Work out the finished part from the listing and answer in its coordinate system (mm). Face numbers are marked on the shaded views. Round coordinates to 2 decimals unless told otherwise and drop trailing zeros. Loops run counter-clockwise (first coordinate to the right, second up) from the corner with the lowest first, then second, coordinate; pieces in that order, holes last. Notation, with made-up numbers: (47, 54.25) -> (86, 54.25) arc R33 ccw to (86, 83.25) -> close; hole circle Ø1 at (27.5, 79). An arc over 180 degrees is marked (long way). Use one line per item in the form item = value.
```python
from build123d import *

# Parameters (mm, degrees)
F0_W     = 25.4
F0_H     = 25.4
F0_W_2   = 22.225
F0_H_2   = 22.225
F1_DEPTH = 292.1
F3_DEPTH = 25.401
F5_DEPTH = 25.401


with BuildPart() as f1:
    # F0 (on Front) → F1 (new body, symmetric)
    with BuildSketch(Plane.XZ):
        Rectangle(F0_W, F0_H)
        Rectangle(F0_W_2, F0_H_2, mode=Mode.SUBTRACT)
    extrude(amount=F1_DEPTH, both=True)

    # F2 (on face) → F3 (cut, through all)
    with BuildSketch(Plane.XY.offset(12.7)):
        Polygon((12.7, 292.1), (-12.7, 292.1), (-12.7, 287.621295), align=None)
    extrude(amount=-F3_DEPTH, mode=Mode.SUBTRACT)

    # F4 (on face) → F5 (cut, through all)
    with BuildSketch(Plane.XY.offset(12.7)):
        Polygon((12.7, -287.621295), (-12.7, -292.1), (12.7, -292.1), align=None)
    extrude(amount=-F5_DEPTH, mode=Mode.SUBTRACT)


solid = f1.part
```
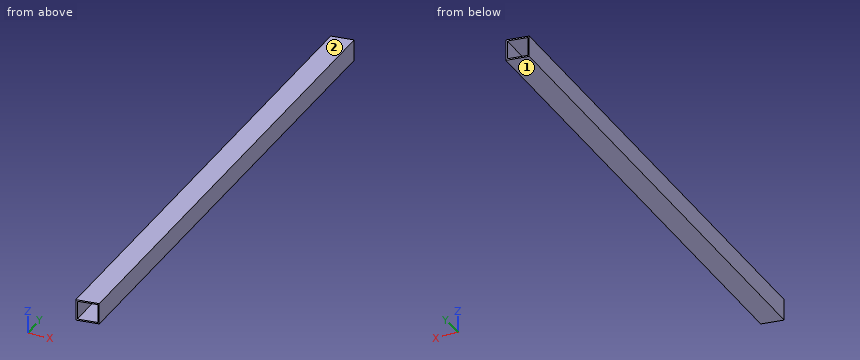
(1) Consider L1, parallel to Z at x = -10.5, y = -87. Determine where the line is inside the solid, lowest interval first.
Completed:
L1 = -12.7 to -11.11, 11.11 to 12.7
(2) For a pull along Z with two mould halves and no side action, classify the marked faces 1 and 2 as +Z half, -Z half, draft (parallel to the pull), parting line (faces both ways), or undercut.
Completed:
face_1 = -Z half
face_2 = +Z half
(3) Find section A-A, the plane y = 118.5. Write down the section's boundary in (x, z), then the cut area to 3 significant figures.
Completed:
outline = (-12.7, -12.7) -> (12.7, -12.7) -> (12.7, 12.7) -> (-12.7, 12.7) -> close; hole (-11.11, -11.11) -> (11.11, -11.11) -> (11.11, 11.11) -> (-11.11, 11.11) -> close
area = 151 mm2
(4) Find section B-B, the plane x = -6.25. Write down the section's boundary in (y, z).
Completed:
outline = (-290.96, -12.7) -> (288.76, -12.7) -> (288.76, -11.11) -> (-290.96, -11.11) -> close; (-290.96, 11.11) -> (288.76, 11.11) -> (288.76, 12.7) -> (-290.96, 12.7) -> close
